Here's how the part is built. I have some questions about the finished solid (model axes, mm). A direction names the side the tool comes from. Round coordinates to 2 decimals unless told otherwise and drop trailing zeros. Order: outer loops, then holes, each group sorted by start corner. A loop starts at its lowest first (then second) coordinate and runs counter-clockwise, first axis right, second up. Notation, with made-up numbers: (14, 38) - (65, 38) arc R28 cw to (65, 71) - close; hole circle Ø3 at (-38, 67). An arc over 180 degrees is marked (long way). One line per item, written item: value.
from build123d import *

# Parameters (mm, degrees)
BOSS_EXTRUDE1_DEPTH = 44.45
SKETCH2_R           = 3.175
CUT_EXTRUDE1_DEPTH  = 73.122135992


with BuildPart() as part:
    # Sketch1 → Boss-Extrude1 (new body)
    with BuildSketch(Plane(origin=(0, 0, 0), x_dir=(1, 0, 0), z_dir=(0, 1, 0))):
        Polygon((47.625, 25.4), (50.8, 25.4), (50.8, 0), (0, 0), (0, 25.4), (3.175, 25.4), (3.175, 3.175), (47.625, 3.175), align=None)
    extrude(amount=BOSS_EXTRUDE1_DEPTH)

    # Sketch2 → Cut-Extrude1 (cut, through all)
    with BuildSketch(Plane.XY):
        with Locations((25.4, 22.225)):
            Circle(SKETCH2_R)
    extrude(amount=-CUT_EXTRUDE1_DEPTH, mode=Mode.SUBTRACT)


solid = part.part
Q1. If we section it at A-A, the plane z = -11.5: Please give me the cut outline in (x, y) (3 decimals), then the cut area to 3 significant figures.
Results list:
outline: (0, 0) - (3.175, 0) - (3.175, 44.45) - (0, 44.45) - close; (47.625, 0) - (50.8, 0) - (50.8, 44.45) - (47.625, 44.45) - close
area: 282 mm²
Q2. Which directions (+Z, -Z, +X, -X, +Y, -Y) give clear straight access to the entire face, cutting with the end or side of a thin tool? Please do faces 1 (the cylindrical face through (28.43, 23.18, -1.57)), 2 (the flat face through (47.625, 22, -14)).
Results list:
face 1: +Z, -Z
face 2: -Z, +Y, -Y
Q3. Will these pins go through, and if not, where does the flat tip stop? pin 1 (4 mm diameter, centred on x = 5.5, z = -12, fed in from -Y); pin 2 (10 mm diameter, centred on x = 25.4, y = 22.225, fed in from -Z) (3 decimals).
Results list:
pin 1: through
pin 2: z = -3.175
Q4. If I drill on line 1 along X through (y, z) = (6.5, -13) (3 decimals); line 2 along Y through (x, z) = (25.4, -1.3); line 3 along Z through (x, y) = (28.5, 20) (3 decimals), over which ranges is the centre line in solid material (lowest first)?
Results list:
line 1: 0 to 3.175, 47.625 to 50.8
line 2: 0 to 19.05, 25.4 to 44.45
line 3: -3.175 to 0
Q5. If we section it at B-B, the plane x = 25.4: Please give me the cut outline in (y, z) (3 decimals), then the cut area to 3 significant figures.
Results list:
outline: (0, -3.175) - (19.05, -3.175) - (19.05, 0) - (0, 0) - close; (25.4, -3.175) - (44.45, -3.175) - (44.45, 0) - (25.4, 0) - close
area: 121 mm²
Q6. If we section it at C-C, the plane y = 36: Please give me the cut outline in (x, z) (3 decimals).
Results list:
outline: (0, -25.4) - (3.175, -25.4) - (3.175, -3.175) - (47.625, -3.175) - (47.625, -25.4) - (50.8, -25.4) - (50.8, 0) - (0, 0) - close
Q7. If we section it at D-D, the plane x = 12: Please give me the cut outline in (y, z) (3 decimals), then the cut area to 3 significant figures.
Results list:
outline: (0, -3.175) - (44.45, -3.175) - (44.45, 0) - (0, 0) - close
area: 141 mm²
